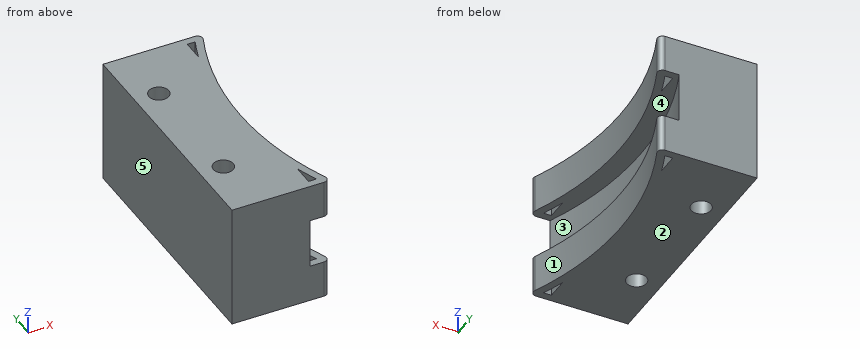
```python
from build123d import *

# Parameters (mm, degrees)
F0_W     = 14.641710973
F0_H     = 25
F0_R     = 2
F2_DEPTH = 25
F1_W     = 8
F1_H     = 10
F4_R     = 1


# Not quite as in the source:
# - a feature names something its author has since deleted; it is built from what else it names


with BuildPart() as f2:
    # F0 (on Top) → F2 (new body)
    with BuildSketch(Plane.XY):
        with BuildLine():
            ThreePointArc((-61, 0), (-59.6453869522, 12.7838888967), (-55.641710973, 25))
            Line((-55.641710973, 25), (-61, 25))
            Line((-61, 25), (-61, 0))
        make_face()
        with BuildLine():
            Line((-59.5, 19.1311264697), (-59.5, 23.5))
            Line((-59.5, 23.5), (-57.9137289423, 23.5))
            ThreePointArc((-57.9137289423, 23.5), (-58.7474910104, 21.3303141089), (-59.5, 19.1311264697))
        make_face(mode=Mode.SUBTRACT)
        with BuildLine():
            ThreePointArc((-55.641710973, -25), (-59.6453869522, -12.7838888967), (-61, 0))
            Line((-61, 0), (-61, -25))
            Line((-61, -25), (-55.641710973, -25))
        make_face()
        with BuildLine():
            Line((-57.9137289423, -23.5), (-59.5, -23.5))
            Line((-59.5, -23.5), (-59.5, -19.1311264697))
            ThreePointArc((-59.5, -19.1311264697), (-58.7474910104, -21.3303141089), (-57.9137289423, -23.5))
        make_face(mode=Mode.SUBTRACT)
        with Locations((-68.3208554865, -12.5)):
            Rectangle(F0_W, F0_H)
        with Locations((-70.891710973, -12.5)):
            Circle(F0_R, mode=Mode.SUBTRACT)
        with Locations((-68.3208554865, 12.5)):
            Rectangle(F0_W, F0_H)
        with Locations((-70.891710973, 12.5)):
            Circle(F0_R, mode=Mode.SUBTRACT)
    extrude(amount=F2_DEPTH)

    # F1 (on Front) → F3 (revolve, cut)
    with BuildSketch(Plane.XZ):
        with Locations((-61, 12.5)):
            Rectangle(F1_W, F1_H)
    revolve(axis=Axis((0, 0, 15.2043728158), (0, 0, 1)), mode=Mode.SUBTRACT)

    # F4
    f4_edges = [f2.edges().sort_by_distance(p)[0] for p in [
        (-55.641711, 25, 21.25),
        (-55.641711, 25, 3.75),
        (-55.641711, -25, 3.75),
        (-55.641711, -25, 21.25),
    ]]
    fillet(f4_edges, radius=F4_R)


solid = f2.part
```
Geometry check sheet. Reference: the model listing, model coordinates, mm. Face numbers are marked on the shaded views. A direction names the side the tool comes from. Coordinates: 2 decimals unless noted, no trailing zeros. Loops run counter-clockwise (first coordinate to the right, second up) from the corner with the lowest first, then second, coordinate; pieces in that order, holes last. Notation, with made-up numbers: (62.25, -35.75) - (104.25, -35.75) arc R27 ccw to (104.25, -0.75) - close; hole circle Ø1 at (19.5, 79). An arc over 180 degrees is marked (long way). One line per item, written item: value. Start each with the question number.
(1) Material ranges on line 1 (Z direction, x = -62.25, y = -12); line 2 (Y direction, x = -72.5, z = 19.5); line 3 (Y direction, x = -69.5, z = 7), recorded low to high. Write a range as [from, to].
(2) Depth check by flat-ended pin: P1, Ø3.5, axis at y = -21, z = 2, coming from the +X side; P2, Ø3, axis at x = -70.89, y = 12.5, coming from the +Z side; P3, Ø3.5, axis at y = 22, z = 2.5, coming from the +X side; P4, Ø1.3, axis at y = 20.5, z = 20.5, coming from the +X side. Enter the tip coordinate at first touch or a pass-through.
(3) Tool access check on the marked faces 4 and 5. Record the directions out of +Z, -Z, +X, -X, +Y, -Y that give a thin tool (end or side, any length) a straight path to the whole face; none if there is none.
(4) Cross-section at A-A on z = 18.25. Enter the section's corners in (x, y).
(5) Cross-section at C-C on y = -11. Enter the section's corners in (x, z).
(6) Cross-section at D-D on y = -4.5. Enter the section's corners in (x, z), plus the area to 3 significant figures.
(7) Cross-section at B-B on z = 9.25. Enter the section's corners in (x, y), plus the area to 3 significant figures.
(8) Mould release check, pull along Z, two halves, no side actions. Record for the marked faces 1, 2 and 3: released by +Z, released by -Z, zero draft, split by the parting line, or undercut.
Results below:
1. line 1: z = [0, 7.5], [17.5, 25]
1. line 2: y = [-25, -13.69], [-11.31, 11.31], [13.69, 25]
1. line 3: y = [-25, -13.94], [-11.06, 11.06], [13.94, 25]
2. P1: stops at x = -56.6
2. P2: passes through
2. P3: stops at x = -56.2
2. P4: stops at x = -57.22
3. face 4: +X
3. face 5: +Z, -Z, -X, +Y, -Y
4. outline: (-75.64, -25) - (-57.17, -25) arc R1 ccw to (-56.24, -23.61) arc R61 cw to (-56.24, 23.61) arc R1 ccw to (-57.17, 25) - (-75.64, 25) - close; hole circle Ø4 at (-70.89, -12.5); hole circle Ø4 at (-70.89, 12.5); hole (-59.5, -23.5) - (-57.91, -23.5) arc R62.5 cw to (-59.5, -19.13) - close; hole (-59.5, 19.13) arc R62.5 cw to (-57.91, 23.5) - (-59.5, 23.5) - close
5. outline: (-75.64, 0) - (-72.21, 0) - (-72.21, 25) - (-75.64, 25) - close; (-69.57, 0) - (-60, 0) - (-60, 7.5) - (-64.06, 7.5) - (-64.06, 17.5) - (-60, 17.5) - (-60, 25) - (-69.57, 25) - close
6. outline: (-75.64, 0) - (-60.83, 0) - (-60.83, 7.5) - (-64.84, 7.5) - (-64.84, 17.5) - (-60.83, 17.5) - (-60.83, 25) - (-75.64, 25) - close
6. area: 330 mm2
7. outline: (-75.64, -25) - (-60, -25) arc R65 cw to (-60, 25) - (-75.64, 25) - close; hole circle Ø4 at (-70.89, -12.5); hole circle Ø4 at (-70.89, 12.5)
7. area: 589 mm2
8. face 1: zero draft
8. face 2: released by -Z
8. face 3: undercut
